Input: dimensioned drawing with shaded views. Units: mm. Origin: part minimum x, y, z. A direction names the side the tool comes from. Give positions to 0.01 mm unless a question says otherwise; leave off trailing zeros. Write each loop counter-clockwise with the first axis right and the second up, starting at its lowest first coordinate (ties: lowest second). Pieces come first, ordered by that corner, then holes.
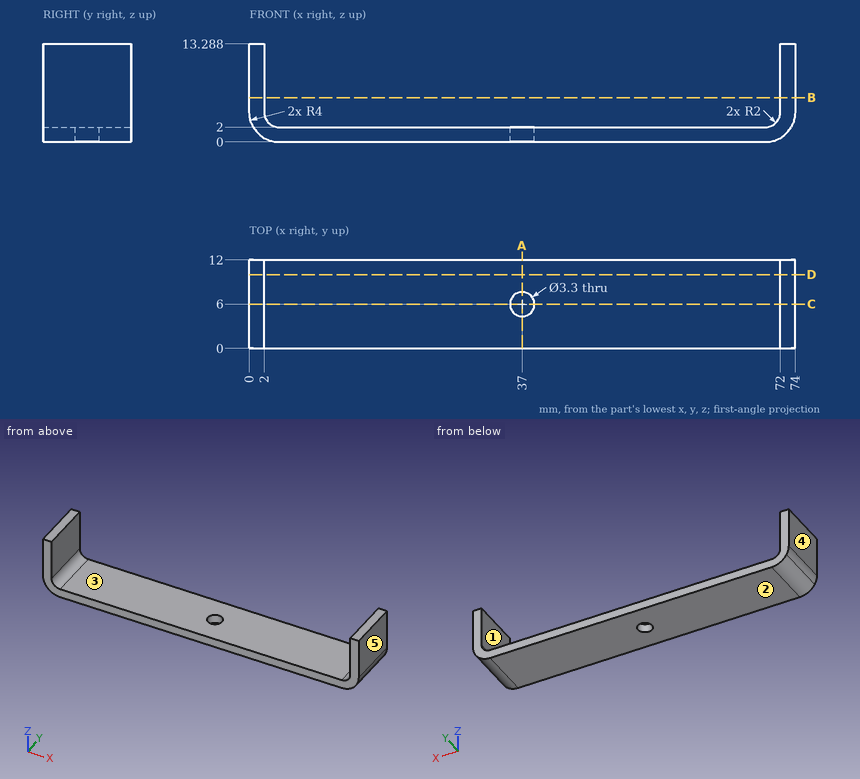
Item 1: Pin query (flat end, axial travel): pin 1 (2 mm diameter, centred on x = 25.5, y = 10, fed in from +Z). Return the tip coordinate at first contact, or that it passes through.
Item 2: Ray query, line 1 (X direction, y = 9.75, z = 8.75); line 2 (Y direction, x = 37, z = 1.2); line 3 (Z direction, x = 32, y = 2.25). Return the intervals inside material, ascending.
Item 3: Mould query, pull axis X, two halves, no side actions, for the marked faces 3, 4 and 5. Classes: +X half, -X half, draft (parallel to the pull), parting line (faces both ways), or undercut.
Item 4: Section D-D (y = 10). Return loops of the section in (x, z).
Item 5: Section A-A (x = 37). Return loops of the section in (y, z).
Item 6: Section C-C (y = 6). Return loops of the section in (x, z).
Item 7: Section B-B (z = 6). Return loops of the section in (x, y).
Item 8: Set-up query: the marked faces 1 and 2. Return all of +Z, -Z, +X, -X, +Y, -Y with unobstructed straight access to the full face (end or side cutting, diameter ignored); none if empty.
Solved:
1. pin 1: stops at z = 2
2. line 1: x = 0 to 2, 72 to 74
2. line 2: y = 0 to 4.35, 7.65 to 12
2. line 3: z = 0 to 2
3. face 3: undercut
3. face 4: -X half
3. face 5: +X half
4. outline: (0, 4) arc R4 ccw to (4, 0) - (70, 0) arc R4 ccw to (74, 4) - (74, 13.29) - (72, 13.29) - (72, 4) arc R2 cw to (70, 2) - (4, 2) arc R2 cw to (2, 4) - (2, 13.29) - (0, 13.29) - close
5. outline: (0, 0) - (4.35, 0) - (4.35, 2) - (0, 2) - close; (7.65, 0) - (12, 0) - (12, 2) - (7.65, 2) - close
6. outline: (0, 4) arc R4 ccw to (4, 0) - (35.35, 0) - (35.35, 2) - (4, 2) arc R2 cw to (2, 4) - (2, 13.29) - (0, 13.29) - close; (38.65, 0) - (70, 0) arc R4 ccw to (74, 4) - (74, 13.29) - (72, 13.29) - (72, 4) arc R2 cw to (70, 2) - (38.65, 2) - close
7. outline: (0, 0) - (2, 0) - (2, 12) - (0, 12) - close; (72, 0) - (74, 0) - (74, 12) - (72, 12) - close
8. face 1: +Z, +Y, -Y
8. face 2: -Z, +X, -X, +Y, -Y
